Model file for the job. Use its own axes, mm. A direction names the side the tool comes from. Coordinates: 2 decimals unless noted, no trailing zeros. Order: outer loops, then holes, each group sorted by start corner. A loop starts at its lowest first (then second) coordinate and runs counter-clockwise, first axis right, second up. Notation, with made-up numbers: (-2, 13.25) - (37, 13.25) arc R28 ccw to (37, 33.25) - close; hole circle Ø9 at (-15.75, -7.5). An arc over 180 degrees is marked (long way). Put each result on its own line as item: value. Start each with the question number.
```python
from build123d import *

# Parameters (mm, degrees)
SKETCH1_R           = 1.4
BOSS_EXTRUDE1_DEPTH = 2


with BuildPart() as part:
    # Sketch1 → Boss-Extrude1 (new body)
    with BuildSketch(Plane.XY):
        with BuildLine():
            Line((-1.5, -3.4), (-1.5, -1.4))
            Line((-1.5, -1.4), (-3.5, -1.4))
            Line((-3.5, -1.4), (-3.5, 3.6))
            Line((-3.5, 3.6), (-1.5, 3.6))
            Line((-1.5, 3.6), (-1.5, 11.6))
            Line((-1.5, 11.6), (3.099578521, 1.397359292))
            ThreePointArc((3.099578521, 1.397359292), (2.855785495, -1.845125796), (0, -3.4))
            Line((0, -3.4), (-1.5, -3.4))
        make_face()
        Circle(SKETCH1_R, mode=Mode.SUBTRACT)
    extrude(amount=BOSS_EXTRUDE1_DEPTH)


solid = part.part
```
Item 1: Slice it at B-B, the plane z = 1.6. Give the cut face in (x, y).
Item 2: Wall check: line 1 along Y through (x, z) = (1, 1.8); line 2 along Y through (x, z) = (-2.25, 1.6); line 3 along Y through (x, z) = (0, 0.8). Give the ranges that are in metal, low to high.
Item 3: Slice it at A-A, the plane y = 0. Give the cut face in (x, z).
Item 4: 3-axis set-ups, long thin cutter, end or side, ignore diameter. For faces 4 (the face through (-1.5, -2, 1)), 5 (the face through (0, 3, 2)), 6 (the face through (-1.5, 8, 1)): which of +Z, -Z, +X, -X, +Y, -Y reach the whole face in a straight line?
Item 5: Slice it at D-D, the plane x = -3. Give the cut face in (y, z).
Item 6: Pull direction Y, two halves, no side cores. Call faces 1 (the face through (-2, -1.4, 1)), 2 (the face through (-3.5, 1, 1)), 3 (the face through (-1.4, 0.06, 0.99)): pulls with the +Y half, pulls with the -Y half, needs draft (parallel to the pull), parting line crosses it, or undercut.
Item 7: Slice it at C-C, the plane x = 0.75. Give the cut face in (y, z).
Item 8: Flat gauge pin, fed straight in: pin 1 Ø0.6 at (y, z) = (-3, 1) entering from -X. Where does the tip first touch, or does it go through?
Here are the results:
1. outline: (-3.5, -1.4) - (-1.5, -1.4) - (-1.5, -3.4) - (0, -3.4) arc R3.4 ccw to (3.1, 1.4) - (-1.5, 11.6) - (-1.5, 3.6) - (-3.5, 3.6) - close; hole circle Ø2.8 at (0, 0)
2. line 1: y = -3.25 to -0.98, 0.98 to 6.05
2. line 2: y = -1.4 to 3.6
2. line 3: y = -3.4 to -1.4, 1.4 to 8.27
3. outline: (-3.5, 0) - (-1.4, 0) - (-1.4, 2) - (-3.5, 2) - close; (1.4, 0) - (3.4, 0) - (3.4, 2) - (1.4, 2) - close
4. face 4: +Z, -Z, -X, -Y
4. face 5: +Z, +X, -X, +Y, -Y
4. face 6: +Z, -Z, -X, +Y
5. outline: (-1.4, 0) - (3.6, 0) - (3.6, 2) - (-1.4, 2) - close
6. face 1: pulls with the -Y half
6. face 2: needs draft
6. face 3: undercut
7. outline: (-3.32, 0) - (-1.18, 0) - (-1.18, 2) - (-3.32, 2) - close; (1.18, 0) - (6.61, 0) - (6.61, 2) - (1.18, 2) - close
8. pin 1: stops at x = -1.5
